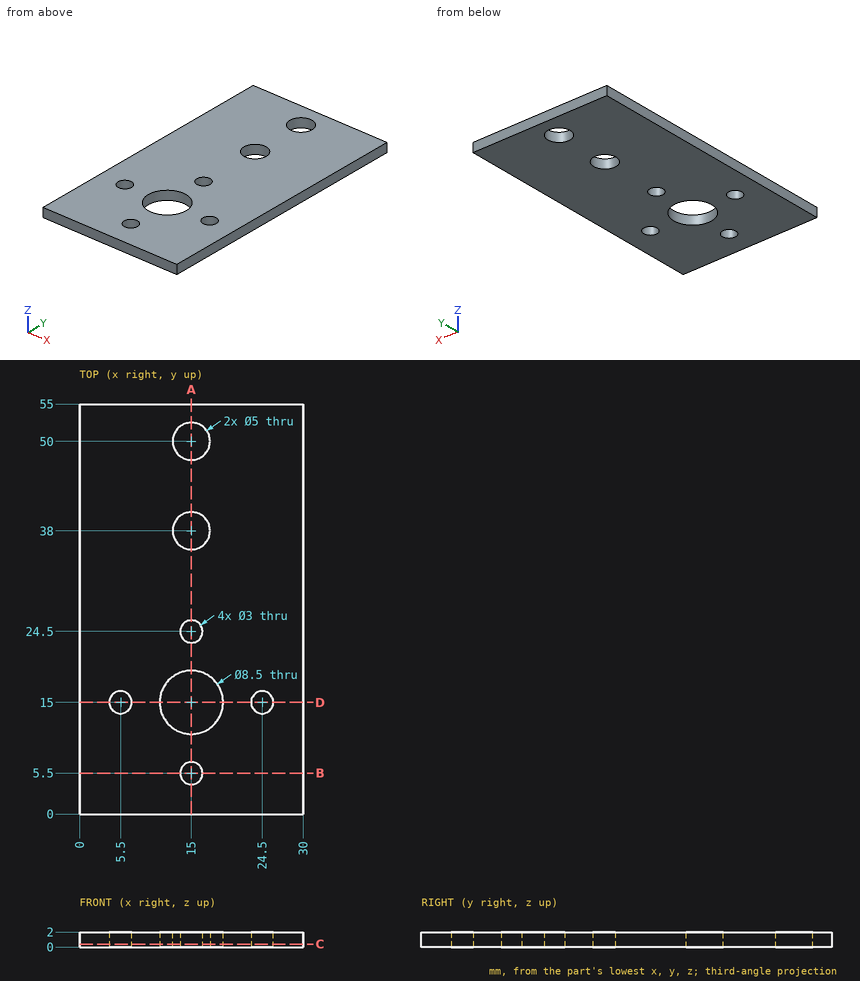
Job drawing, mm, ordinate dimensions from the low corner. One solid piece. Coordinates: 2 decimals unless noted, no trailing zeros. Write each loop counter-clockwise with the first axis right and the second up, starting at its lowest first coordinate (ties: lowest second). Pieces come first, ordered by that corner, then holes.
Item 1: Slice it at B-B (y = 5.5). Write the cut outline in (x, z), and give its area (3 significant figures).
Item 2: Slice it at C-C (z = 0.4). Write the cut outline in (x, y), and give its area (3 significant figures).
Item 3: Probe line 1 (Y direction, x = 15, z = 1); line 2 (Y direction, x = 23.25, z = 0.15); line 3 (Y direction, x = 13, z = 1.3). List the from-to ranges inside material, lowest first.
Item 4: Slice it at A-A (x = 15). Write the cut outline in (y, z).
Item 5: Slice it at D-D (y = 15). Write the cut outline in (x, z), and give its area (3 significant figures).
Results found:
1. outline: (0, 0) - (13.5, 0) - (13.5, 2) - (0, 2) - close; (16.5, 0) - (30, 0) - (30, 2) - (16.5, 2) - close
1. area: 54.0 mm2
2. outline: (0, 0) - (30, 0) - (30, 55) - (0, 55) - close; hole circle Ø3 at (5.5, 15); hole circle Ø8.5 at (15, 15); hole circle Ø5 at (15, 38); hole circle Ø5 at (15, 50); hole circle Ø3 at (15, 5.5); hole circle Ø3 at (15, 24.5); hole circle Ø3 at (24.5, 15)
2. area: 1,530 mm2
3. line 1: y = 0 to 4, 7 to 10.75, 19.25 to 23, 26 to 35.5, 40.5 to 47.5, 52.5 to 55
3. line 2: y = 0 to 14.17, 15.83 to 55
3. line 3: y = 0 to 11.25, 18.75 to 36.5, 39.5 to 48.5, 51.5 to 55
4. outline: (0, 0) - (4, 0) - (4, 2) - (0, 2) - close; (7, 0) - (10.75, 0) - (10.75, 2) - (7, 2) - close; (19.25, 0) - (23, 0) - (23, 2) - (19.25, 2) - close; (26, 0) - (35.5, 0) - (35.5, 2) - (26, 2) - close; (40.5, 0) - (47.5, 0) - (47.5, 2) - (40.5, 2) - close; (52.5, 0) - (55, 0) - (55, 2) - (52.5, 2) - close
5. outline: (0, 0) - (4, 0) - (4, 2) - (0, 2) - close; (7, 0) - (10.75, 0) - (10.75, 2) - (7, 2) - close; (19.25, 0) - (23, 0) - (23, 2) - (19.25, 2) - close; (26, 0) - (30, 0) - (30, 2) - (26, 2) - close
5. area: 31.0 mm2
